Solid Edge part; units mm, degrees
sketch "Sketch1" plane through (0, 0, 0) normal (0, -1, 0) x (1, 0, 0)
  line L0 (-95, 139.7) -> (-95, 68.5)
  line L1 (-95, 68.5) -> (-90, 68.5)
  line L2 (-90, 68.5) -> (-90, 63.5)
  line L3 (-90, 63.5) -> (-80, 63.5)
  line L4 (-80, 63.5) -> (-80, 68.5)
  line L5 (-80, 68.5) -> (-85, 68.5)
  line L6 (-85, 68.5) -> (-85, 73.5)
  line L7 (-85, 73.5) -> (-90, 73.5)
  line L8 (-90, 73.5) -> (-90, 134.7)
  line L9 (-90, 134.7) -> (90, 134.7)
  line L10 (90, 134.7) -> (90, 73.5)
  line L11 (90, 73.5) -> (85, 73.5)
  line L12 (85, 73.5) -> (85, 68.5)
  line L13 (85, 68.5) -> (80, 68.5)
  line L14 (80, 68.5) -> (80, 63.5)
  line L15 (80, 63.5) -> (90, 63.5)
  line L16 (90, 63.5) -> (90, 68.5)
  line L17 (90, 68.5) -> (95, 68.5)
  line L18 (95, 68.5) -> (95, 139.7)
  line L19 (95, 139.7) -> (-95, 139.7)
  dimension "D1" = 90
  dimension "D2" = 80
  dimension "D3" = 85
  dimension "D4" = 80
  dimension "D5" = 80
  dimension "D6" = 85
  dimension "D7" = 90
  dimension "D8" = 85
  dimension "D9" = 90
revolve "RevolvedProtrusion1" add sketch "Sketch1" angle 360 about axis through (-79.3986, 0, 0) along (1, 0, 0)
fillet "Round1" radius 5 4 edges at (95, 0, -139.7) (90, 0, -134.7) (-95, 0, -139.7) (-90, 0, -134.7)
properties material "Phenolic"
Geometry check sheet. Reference: the model listing, model coordinates, mm. A direction names the side the tool comes from. Round coordinates to 2 decimals unless told otherwise and drop trailing zeros. Order: outer loops, then holes, each group sorted by start corner. A loop starts at its lowest first (then second) coordinate and runs counter-clockwise, first axis right, second up. Notation, with made-up numbers: (32, -8.5) - (41, -8.5) arc R25 cw to (41, 4.5) - close; hole circle Ø6 at (87.5, 89). An arc over 180 degrees is marked (long way). Use a Markdown table: item, result. Add a question column.
(1) Material ranges on line 1 along Z through (x, y) = (84, 0); line 2 along Z through (x, y) = (-85.5, 0), recorded low to high. Write a range as [from, to].
(2) Sectioned sample at A-A, the plane x = 55.5. Enter the section's corners in (y, z), and give its area (3 significant figures).
(3) Tool access check on faces 1 (the cylindrical face through (-92.465, -20.576, 65.337)), 2 (the flat face through (90, 61, 20)), 3 (the cylindrical face through (-84.93, 61.99, -13.77)), 4 (the flat face through (-90, 56, 56)). Record the directions out of +Z, -Z, +X, -X, +Y, -Y that give a thin tool (end or side, any length) a straight path to the whole face; none if there is none.
(4) Depth check by flat-ended pin: pin 1 (3 mm diameter, centred on x = -38, z = 31, fed in from +Y); pin 2 (5 mm diameter, centred on x = -70.5, y = -59, fed in from -Z); pin 3 (10 mm diameter, centred on y = 67.5, z = 3.5, fed in from -X); pin 4 (8 mm diameter, centred on x = -21.5, y = -86.5, fed in from -Z). Enter the tip coordinate at first touch or a pass-through.
(5) Release check for a two-part mould opening along Y. For faces 5 (the cylindrical face through (85.07, 61.99, -13.77)), 6 (the flat face through (-95, -32, -62)), 7 (the cylindrical face through (-1.26, -85.01, -110.86)) record: pulls with the +Y half, pulls with the -Y half, needs draft (parallel to the pull), parting line crosses it, or undercut.
Answers below:
| question | item | result |
|---|---|---|
| 1 | line 1 | [-139.7, -134.7], [-68.5, -63.5], [63.5, 68.5], [134.7, 139.7] |
| 1 | line 2 | [-139.7, -134.67], [-73.5, -63.5], [63.5, 73.5], [134.67, 139.7] |
| 2 | outline | circle Ø279.4 at (0, 0); hole circle Ø269.4 at (0, 0) |
| 2 | area | 4,310 mm² |
| 3 | face 1 | -X |
| 3 | face 2 | +X |
| 3 | face 3 | +X, -X |
| 3 | face 4 | none |
| 4 | pin 1 | y = 136.55 |
| 4 | pin 2 | z = -127.76 |
| 4 | pin 3 | x = -95 |
| 4 | pin 4 | z = -112.74 |
| 5 | face 5 | undercut |
| 5 | face 6 | needs draft |
| 5 | face 7 | parting line crosses it |
